Autodesk Inventor part; units mm, degrees
ref_plane "ANBAU_XY" through (0, 0, 0) normal (0, 1, 0) x (1, 0, 0)
ref_plane "ANBAU_YZ" through (0, 0, 0) normal (1, 0, 0) x (0, 0, -1)
ref_plane "ANBAU_ZX" through (0, 0, 0) normal (0, 0, -1) x (0, 1, 0)
sketch "Sketch_1" plane through (0, 0, 0) normal (0, 0, 1) x (1, 0, 0)
  line L0 (0, -35) -> (0, 10)
  line L1 (0, 2.6906) -> (4, 5)
  line L2 (4, 5) -> (4, 9.3812)
  line L3 (4, 9.3812) -> (4.6188, 10)
  line L4 (4.6188, 10) -> (7, 10)
  line L5 (7, 10) -> (8, 9)
  line L6 (8, 9) -> (8, 0.25)
  line L7 (8, 0.25) -> (7.75, 0)
  line L8 (7.75, 0) -> (5.05, 0)
  line L9 (5.05, 0) -> (5, -1.02)
  line L10 (5, -1.02) -> (5, -34.08)
  line L11 (5, -34.08) -> (4.08, -35)
  line L12 (4.08, -35) -> (0, -35)
  line L13 (0, -35) -> (0, 2.6906)
revolve "Revolution1" add sketch "Sketch_1" angle 360 about axis through (0, -35, 0) along (0, -1, 0)
thread "Thread1"
sketch "Sketch_2" plane through (0, 10, 0) normal (0, 1, 0) x (1, 0, 0)
  line L0 (-4, -2.3094) -> (0, -4.6188)
  line L1 (0, -4.6188) -> (4, -2.3094)
  line L2 (4, -2.3094) -> (4, 2.3094)
  line L3 (4, 2.3094) -> (0, 4.6188)
  line L4 (0, 4.6188) -> (-4, 2.3094)
  line L5 (-4, 2.3094) -> (-4, -2.3094)
extrude "Extrusion1" cut sketch "Sketch_2" against normal blind 5
ref_plane "ANBAU_XY" through (0, 0, 0) normal (0, 1, 0) x (1, 0, 0)
ref_plane "ANBAU_YZ" through (0, 0, 0) normal (1, 0, 0) x (0, 0, -1)
ref_plane "ANBAU_ZX" through (0, 0, 0) normal (0, 0, -1) x (0, 1, 0)
ref_plane "Schraube_XY" through (0, 0, 0) normal (0, 1, 0) x (1, 0, 0)
ref_plane "Schraube_YZ" through (0, 0, 0) normal (1, 0, 0) x (0, 0, -1)
ref_plane "Schraube_ZX" through (0, 0, 0) normal (0, 0, -1) x (0, 1, 0)
ref_plane "insert_XY" through (0, 0, 0) normal (0, 1, 0) x (1, 0, 0)
ref_plane "insert_YZ" through (0, 0, 0) normal (1, 0, 0) x (0, 0, -1)
ref_plane "insert_ZX" through (0, 0, 0) normal (0, 0, -1) x (0, 1, 0)
ref_plane "schrauben_punkt_XY" through (0, -35, 0) normal (0, 1, 0) x (1, 0, 0)
ref_plane "schrauben_punkt_YZ" through (0, -35, 0) normal (1, 0, 0) x (0, 0, -1)
ref_plane "schrauben_punkt_ZX" through (0, -35, 0) normal (0, 0, -1) x (0, 1, 0)
properties part number "DIN-912 - M10x35(F)"
Design review of the part built by this model. Coordinates are the model's own, in mm. A direction names the side the tool comes from. Coordinates: 2 decimals unless noted, no trailing zeros. Order: outer loops, then holes, each group sorted by start corner. A loop starts at its lowest first (then second) coordinate and runs counter-clockwise, first axis right, second up. Notation, with made-up numbers: (-22.75, 4.25) -> (19.25, 4.25) arc R21 cw to (19.25, 22.25) -> close; hole circle Ø3 at (29.25, 32). An arc over 180 degrees is marked (long way). One line per item, written item: value. Start each with the question number.
Q1. Insertion check: pin 1 Ø0.6 at (x, z) = (2.5, -1) entering from +Y; pin 2 Ø4 at (y, z) = (-20, -4.5) entering from +X; pin 3 Ø6 at (x, y) = (-3.5, -22.5) entering from -Z; pin 4 Ø1.5 at (x, y) = (-6, -28.5) entering from +Z. Each pin has a flat end and moves straight along its axis. Give the tip position at first contact, or say it passes through.
Q2. Take a section at A-A, the plane y = -32. State the section outline as (x, z) points.
Q3. For probe 1 along X at (y, z) = (7.5, 2); probe 2 along Y at (x, z) = (-5.25, 1.25); probe 3 along Z at (x, y) = (-2.5, 6), list the stretches that pass through material, from the lowest coordinate up.
Q4. Mouldability with a two-part tool opening along Z and no side actions: class faces 4 (the conical face through (-1.087, -0.73, 4.895)), 5 (the flat face through (0, -35, 0)), 6 (the flat face through (-2.028, 7.535, 3.448)) as pulls with the +Z half, pulls with the -Z half, needs draft (parallel to the pull), parting line crosses it, or undercut.
Q5. Tool access review of faces 1 (the flat face through (2, 0, -5)), 2 (the flat face through (-3.6, 5, -2.1)), 3 (the flat face through (1, 10, -5)): name each direction out of +Z, -Z, +X, -X, +Y, -Y from which nothing blocks a thin tool from reaching the whole face with its end or side.
Values follow:
1. pin 1: stops at y = 4.42
1. pin 2: stops at x = 4.33
1. pin 3: stops at z = -4.97
1. pin 4: passes through
2. outline: circle Ø10 at (0, 0)
3. probe 1: x = -7.75 to -4, 4 to 7.75
3. probe 2: y = 0 to 10
3. probe 3: z = -7.6 to -3.18, 3.18 to 7.6
4. face 4: parting line crosses it
4. face 5: needs draft
4. face 6: undercut
5. face 1: -Y
5. face 2: +Y
5. face 3: +Z, -Z, +X, -X, +Y
